```python
from build123d import *

# Parameters (mm, degrees)
SKETCH1_R               = 30
BOSS_EXTRUDE1_DEPTH     = 25
SKETCH2_R               = 16
CUT_EXTRUDE1_DEPTH      = 25
BOSS_EXTRUDE3_DEPTH     = 25
BOSS_EXTRUDE4_DEPTH     = 7.5
SKETCH4_R               = 10
CUT_EXTRUDE2_DEPTH      = 51
SKETCH5_W               = 25
SKETCH5_H               = 45
CUT_EXTRUDE3_DEPTH      = 31
CUT_EXTRUDE3_DEPTH_BACK = 31


with BuildPart() as part:
    # Sketch1 → Boss-Extrude1 (new body, symmetric)
    with BuildSketch(Plane(origin=(0, 0, 0), x_dir=(0, 0, -1), z_dir=(1, 0, 0))):
        Circle(SKETCH1_R)
    extrude(amount=BOSS_EXTRUDE1_DEPTH, both=True)

    # Sketch2 → Cut-Extrude1 (cut, symmetric)
    with BuildSketch(Plane(origin=(0, 0, 0), x_dir=(0, 0, -1), z_dir=(1, 0, 0))):
        Circle(SKETCH2_R)
    extrude(amount=CUT_EXTRUDE1_DEPTH, both=True, mode=Mode.SUBTRACT)



with BuildPart() as body_2:
    # Sketch3 → Boss-Extrude3 (new body, symmetric)
    with BuildSketch(Plane(origin=(0, 0, 0), x_dir=(0, 0, -1), z_dir=(1, 0, 0))):
        with BuildLine():
            Line((-19.843134833, 82.5), (-25.197631534, 40))
            Line((-25.197631534, 40), (25.197631534, 40))
            Line((25.197631534, 40), (19.843134833, 82.5))
            ThreePointArc((19.843134833, 82.5), (0, 100), (-19.843134833, 82.5))
        make_face()
    extrude(amount=BOSS_EXTRUDE3_DEPTH, both=True)


with BuildPart() as part_1:
    add(part.part)

    add(body_2.part)  # Boss-Extrude4 merges body 2
    # Sketch3<3> → Boss-Extrude4 (add, symmetric)
    with BuildSketch(Plane(origin=(0, 0, 0), x_dir=(0, 0, -1), z_dir=(1, 0, 0))):
        with BuildLine():
            Line((25.197631534, 40), (-25.197631534, 40))
            Line((-25.197631534, 40), (-29.764702249, 3.75))
            ThreePointArc((-29.764702249, 3.75), (0, 30), (29.764702249, 3.75))
            Line((29.764702249, 3.75), (25.197631534, 40))
        make_face()
    extrude(amount=BOSS_EXTRUDE4_DEPTH, both=True)

    # Sketch4 → Cut-Extrude2 (cut, through all)
    with BuildSketch(Plane(origin=(25, 0, 0), x_dir=(0, 0, -1), z_dir=(1, 0, 0))):
        with Locations((0, 80)):
            Circle(SKETCH4_R)
    extrude(amount=-CUT_EXTRUDE2_DEPTH, mode=Mode.SUBTRACT)

    # Sketch5 → Cut-Extrude3 (cut, two sides)
    with BuildSketch(Plane.XY) as cut_extrude3_sk:
        with Locations((0, 77.5)):
            Rectangle(SKETCH5_W, SKETCH5_H)
    extrude(amount=CUT_EXTRUDE3_DEPTH, mode=Mode.SUBTRACT)
    extrude(cut_extrude3_sk.sketch, amount=-CUT_EXTRUDE3_DEPTH_BACK, mode=Mode.SUBTRACT)


solid = part_1.part
```
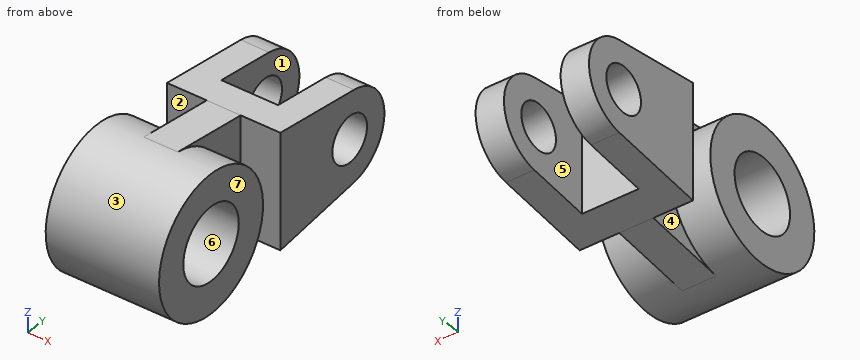
Check sheet for the modelled part. Datum: model origin and axes. Units: mm. Face numbers are marked on the shaded views. A direction names the side the tool comes from. Round coordinates to 2 decimals unless told otherwise and drop trailing zeros. Order: outer loops, then holes, each group sorted by start corner. A loop starts at its lowest first (then second) coordinate and runs counter-clockwise, first axis right, second up. Notation, with made-up numbers: (61, 7.5) -> (101, 7.5) arc R8 cw to (101, 17.5) -> close; hole circle Ø11 at (-39, 42.5). An arc over 180 degrees is marked (long way). One line per item, written item: value. Start each with the question number.
Q1. Gauge pin test, flat ends, axial feed: pin 1 Ø7.5 at (x, z) = (-1.5, -7.5) entering from +Y; pin 2 Ø3 at (x, z) = (7.5, -5) entering from -Y; pin 3 Ø12 at (y, z) = (80, 0) entering from +X; pin 4 Ø9 at (x, z) = (17, 4.5) entering from -Y. Record the tip position at first contact, or that the pin passes through.
Q2. Cross-section at D-D (x = 2). Record the boundary of the cut face in (y, z).
Q3. Cross-section at C-C (y = 6). Record the boundary of the cut face in (x, z).
Q4. Mould release check, pull along X, two halves, no side actions. Record for the marked faces 5, 6 and 7: pulls with the +X half, pulls with the -X half, needs draft (parallel to the pull), parting line crosses it, or undercut.
Q5. Cross-section at A-A (z = 0). Record the boundary of the cut face in (x, y), and give its area (4 significant figures).
Q6. Cross-section at B-B (x = 22.5). Record the boundary of the cut face in (y, z), and give its area (3 significant figures).
Q7. Set-up check for the marked faces 1, 2, 3 and 4: record each of +Z, -Z, +X, -X, +Y, -Y from which the full face is reachable in a straight line by a thin tool's end or side.
Q8. Thickness scan on line 1 (Y direction, x = 18.5, z = -0.5); line 2 (X direction, y = 57.5, z = -13.5); line 3 (Y direction, x = -4, z = 0). Record the ranges inside material, lowest first.
Completed:
1. pin 1: stops at y = 55
1. pin 2: stops at y = -29.8
1. pin 3: passes through
1. pin 4: stops at y = -30
2. outline: (3.75, -29.76) -> (55, -23.31) -> (55, 23.31) -> (3.75, 29.76) arc R30 ccw (long way) to start; hole circle Ø32 at (0, 0)
3. outline: (-25, -29.39) -> (-7.5, -29.39) -> (-7.5, -29.48) -> (7.5, -29.48) -> (7.5, -29.39) -> (25, -29.39) -> (25, -14.83) -> (-25, -14.83) -> close; (-25, 14.83) -> (25, 14.83) -> (25, 29.39) -> (7.5, 29.39) -> (7.5, 29.48) -> (-7.5, 29.48) -> (-7.5, 29.39) -> (-25, 29.39) -> close
4. face 5: undercut
4. face 6: needs draft
4. face 7: pulls with the +X half
5. outline: (-25, -30) -> (25, -30) -> (25, -16) -> (-25, -16) -> close; (-25, 16) -> (25, 16) -> (25, 30) -> (7.5, 30) -> (7.5, 40) -> (25, 40) -> (25, 70) -> (12.5, 70) -> (12.5, 55) -> (-12.5, 55) -> (-12.5, 70) -> (-25, 70) -> (-25, 40) -> (-7.5, 40) -> (-7.5, 30) -> (-25, 30) -> close; (-25, 90) -> (-12.5, 90) -> (-12.5, 100) -> (-25, 100) -> close; (12.5, 90) -> (25, 90) -> (25, 100) -> (12.5, 100) -> close
5. area: 2,925 mm²
6. outline: circle Ø60 at (0, 0); (40, -25.2) -> (82.5, -19.84) arc R20 ccw to (82.5, 19.84) -> (40, 25.2) -> close; hole circle Ø32 at (0, 0); hole circle Ø20 at (80, 0)
6. area: 4,150 mm²
7. face 1: +Z, -Z, +Y
7. face 2: +Z, -Z, -X
7. face 3: none
7. face 4: -X
8. line 1: y = -30 to -15.99, 15.99 to 30, 40 to 70.01, 89.99 to 99.99
8. line 2: x = -25 to -12.5, 12.5 to 25
8. line 3: y = -30 to -16, 16 to 55
